The model under review builds one solid part; all positions refer to its coordinate system, in mm. Coordinates: 2 decimals unless noted, no trailing zeros. Loops run counter-clockwise (first coordinate to the right, second up) from the corner with the lowest first, then second, coordinate; pieces in that order, holes last. Notation, with made-up numbers: M 12.5,3 L 29.5,3 A20 cw 29.5,9 Z; hole C 76.25,13 d5. An arc over 180 degrees is marked long. Write item = value, one per line. Start each with the question number.
Q1. We need section A-A on x = 4.5. Give the boundary of the cut face in (y, z).
Q2. Clearance check with flat-ended pins moving along their axes: pin 1 Ø5.5 at (y, z) = (1066.8, -16.51) entering from +X; pin 2 Ø6 at (y, z) = (473, -20) entering from +X. State where each tip first meets the part, or that it passes through.
Q3. Wall thickness on probe 1 along X at (y, z) = (939.5, -4.5) (3 decimals); probe 2 along Z at (x, y) = (3.25, 67.5); probe 3 along Z at (x, y) = (1.65, 355.6) (3 decimals): over which ranges is each line inside the solid? List them lowest first.
Q4. We need section B-B on y = 227. Give the boundary of the cut face in (x, z) (3 decimals).
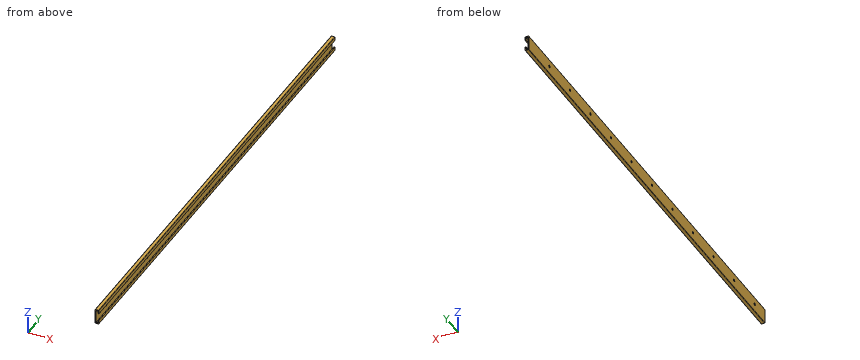
from build123d import *

# Parameters (mm, degrees)
BOSS_EXTRUDE1_DEPTH = 1168.4
CUT_EXTRUDE1_REACH  = 4.54
SKETCH2_R           = 3.175


with BuildPart() as part:
    # Sketch1 → Boss-Extrude1 (new body)
    with BuildSketch(Plane(origin=(0, 0, 0), x_dir=(1, 0, 0), z_dir=(0, 1, 0))):
        with BuildLine():
            Line((9.525, 34.29), (9.525, 26.035))
            Line((9.525, 26.035), (6.985, 26.035))
            Line((6.985, 26.035), (6.985, 33.02))
            Line((6.985, 33.02), (2.54, 33.02))
            Line((2.54, 33.02), (2.54, 0))
            Line((2.54, 0), (6.985, 0))
            Line((6.985, 0), (6.985, 6.985))
            Line((6.985, 6.985), (9.525, 6.985))
            Line((9.525, 6.985), (9.525, -1.27))
            ThreePointArc((9.525, -1.27), (9.153025612, -2.168025612), (8.255, -2.54))
            Line((8.255, -2.54), (1.27, -2.54))
            ThreePointArc((1.27, -2.54), (0.371974388, -2.168025612), (0, -1.27))
            Line((0, -1.27), (0, 34.29))
            ThreePointArc((0, 34.29), (0.371974388, 35.188025612), (1.27, 35.56))
            Line((1.27, 35.56), (8.255, 35.56))
            ThreePointArc((8.255, 35.56), (9.153025612, 35.188025612), (9.525, 34.29))
        make_face()
    extrude(amount=BOSS_EXTRUDE1_DEPTH)

    # Sketch2 → Cut-Extrude1 (cut, up to next)
    with BuildSketch(Plane(origin=(2.54, 0, 0), x_dir=(0, 0, -1), z_dir=(1, 0, 0)), mode=Mode.PRIVATE) as cut_extrude1_sk1:
        with Locations((16.51, 50.8)):
            Circle(SKETCH2_R)
    cut_extrude1_tool1 = extrude(cut_extrude1_sk1.sketch, amount=-CUT_EXTRUDE1_REACH, mode=Mode.PRIVATE) & part.part
    add(cut_extrude1_tool1.solids().sort_by_distance((2.54, 50.8, -16.51))[0], mode=Mode.SUBTRACT)
    # Sketch2 → Cut-Extrude1 (cut, up to next)
    with BuildSketch(Plane(origin=(2.54, 0, 0), x_dir=(0, 0, -1), z_dir=(1, 0, 0)), mode=Mode.PRIVATE) as cut_extrude1_sk2:
        with Locations((16.51, 152.4)):
            Circle(SKETCH2_R)
    cut_extrude1_tool2 = extrude(cut_extrude1_sk2.sketch, amount=-CUT_EXTRUDE1_REACH, mode=Mode.PRIVATE) & part.part
    add(cut_extrude1_tool2.solids().sort_by_distance((2.54, 152.4, -16.51))[0], mode=Mode.SUBTRACT)
    # Sketch2 → Cut-Extrude1 (cut, up to next)
    with BuildSketch(Plane(origin=(2.54, 0, 0), x_dir=(0, 0, -1), z_dir=(1, 0, 0)), mode=Mode.PRIVATE) as cut_extrude1_sk3:
        with Locations((16.51, 254)):
            Circle(SKETCH2_R)
    cut_extrude1_tool3 = extrude(cut_extrude1_sk3.sketch, amount=-CUT_EXTRUDE1_REACH, mode=Mode.PRIVATE) & part.part
    add(cut_extrude1_tool3.solids().sort_by_distance((2.54, 254, -16.51))[0], mode=Mode.SUBTRACT)
    # Sketch2 → Cut-Extrude1 (cut, up to next)
    with BuildSketch(Plane(origin=(2.54, 0, 0), x_dir=(0, 0, -1), z_dir=(1, 0, 0)), mode=Mode.PRIVATE) as cut_extrude1_sk4:
        with Locations((16.51, 355.6)):
            Circle(SKETCH2_R)
    cut_extrude1_tool4 = extrude(cut_extrude1_sk4.sketch, amount=-CUT_EXTRUDE1_REACH, mode=Mode.PRIVATE) & part.part
    add(cut_extrude1_tool4.solids().sort_by_distance((2.54, 355.6, -16.51))[0], mode=Mode.SUBTRACT)
    # Sketch2 → Cut-Extrude1 (cut, up to next)
    with BuildSketch(Plane(origin=(2.54, 0, 0), x_dir=(0, 0, -1), z_dir=(1, 0, 0)), mode=Mode.PRIVATE) as cut_extrude1_sk5:
        with Locations((16.51, 457.2)):
            Circle(SKETCH2_R)
    cut_extrude1_tool5 = extrude(cut_extrude1_sk5.sketch, amount=-CUT_EXTRUDE1_REACH, mode=Mode.PRIVATE) & part.part
    add(cut_extrude1_tool5.solids().sort_by_distance((2.54, 457.2, -16.51))[0], mode=Mode.SUBTRACT)
    # Sketch2 → Cut-Extrude1 (cut, up to next)
    with BuildSketch(Plane(origin=(2.54, 0, 0), x_dir=(0, 0, -1), z_dir=(1, 0, 0)), mode=Mode.PRIVATE) as cut_extrude1_sk6:
        with Locations((16.51, 558.8)):
            Circle(SKETCH2_R)
    cut_extrude1_tool6 = extrude(cut_extrude1_sk6.sketch, amount=-CUT_EXTRUDE1_REACH, mode=Mode.PRIVATE) & part.part
    add(cut_extrude1_tool6.solids().sort_by_distance((2.54, 558.8, -16.51))[0], mode=Mode.SUBTRACT)
    # Sketch2 → Cut-Extrude1 (cut, up to next)
    with BuildSketch(Plane(origin=(2.54, 0, 0), x_dir=(0, 0, -1), z_dir=(1, 0, 0)), mode=Mode.PRIVATE) as cut_extrude1_sk7:
        with Locations((16.51, 660.4)):
            Circle(SKETCH2_R)
    cut_extrude1_tool7 = extrude(cut_extrude1_sk7.sketch, amount=-CUT_EXTRUDE1_REACH, mode=Mode.PRIVATE) & part.part
    add(cut_extrude1_tool7.solids().sort_by_distance((2.54, 660.4, -16.51))[0], mode=Mode.SUBTRACT)
    # Sketch2 → Cut-Extrude1 (cut, up to next)
    with BuildSketch(Plane(origin=(2.54, 0, 0), x_dir=(0, 0, -1), z_dir=(1, 0, 0)), mode=Mode.PRIVATE) as cut_extrude1_sk8:
        with Locations((16.51, 762)):
            Circle(SKETCH2_R)
    cut_extrude1_tool8 = extrude(cut_extrude1_sk8.sketch, amount=-CUT_EXTRUDE1_REACH, mode=Mode.PRIVATE) & part.part
    add(cut_extrude1_tool8.solids().sort_by_distance((2.54, 762, -16.51))[0], mode=Mode.SUBTRACT)
    # Sketch2 → Cut-Extrude1 (cut, up to next)
    with BuildSketch(Plane(origin=(2.54, 0, 0), x_dir=(0, 0, -1), z_dir=(1, 0, 0)), mode=Mode.PRIVATE) as cut_extrude1_sk9:
        with Locations((16.51, 863.6)):
            Circle(SKETCH2_R)
    cut_extrude1_tool9 = extrude(cut_extrude1_sk9.sketch, amount=-CUT_EXTRUDE1_REACH, mode=Mode.PRIVATE) & part.part
    add(cut_extrude1_tool9.solids().sort_by_distance((2.54, 863.6, -16.51))[0], mode=Mode.SUBTRACT)
    # Sketch2 → Cut-Extrude1 (cut, up to next)
    with BuildSketch(Plane(origin=(2.54, 0, 0), x_dir=(0, 0, -1), z_dir=(1, 0, 0)), mode=Mode.PRIVATE) as cut_extrude1_sk10:
        with Locations((16.51, 965.2)):
            Circle(SKETCH2_R)
    cut_extrude1_tool10 = extrude(cut_extrude1_sk10.sketch, amount=-CUT_EXTRUDE1_REACH, mode=Mode.PRIVATE) & part.part
    add(cut_extrude1_tool10.solids().sort_by_distance((2.54, 965.2, -16.51))[0], mode=Mode.SUBTRACT)
    # Sketch2 → Cut-Extrude1 (cut, up to next)
    with BuildSketch(Plane(origin=(2.54, 0, 0), x_dir=(0, 0, -1), z_dir=(1, 0, 0)), mode=Mode.PRIVATE) as cut_extrude1_sk11:
        with Locations((16.51, 1066.8)):
            Circle(SKETCH2_R)
    cut_extrude1_tool11 = extrude(cut_extrude1_sk11.sketch, amount=-CUT_EXTRUDE1_REACH, mode=Mode.PRIVATE) & part.part
    add(cut_extrude1_tool11.solids().sort_by_distance((2.54, 1066.8, -16.51))[0], mode=Mode.SUBTRACT)


solid = part.part
Returned:
q1.outline = M 0,-35.56 L 1168.4,-35.56 L 1168.4,-33.02 L 0,-33.02 Z; M 0,0 L 1168.4,0 L 1168.4,2.54 L 0,2.54 Z
q2.pin_1 = through
q2.pin_2 = 2.54
q3.probe_1 = 0 to 2.54, 6.985 to 9.525
q3.probe_2 = -35.56 to -33.02, 0 to 2.54
q3.probe_3 = -35.56 to -19.685, -13.335 to 2.54
q4.outline = M 0,-34.29 A1.27 ccw 1.27,-35.56 L 8.255,-35.56 A1.27 ccw 9.525,-34.29 L 9.525,-26.035 L 6.985,-26.035 L 6.985,-33.02 L 2.54,-33.02 L 2.54,0 L 6.985,0 L 6.985,-6.985 L 9.525,-6.985 L 9.525,1.27 A1.27 ccw 8.255,2.54 L 1.27,2.54 A1.27 ccw 0,1.27 Z
